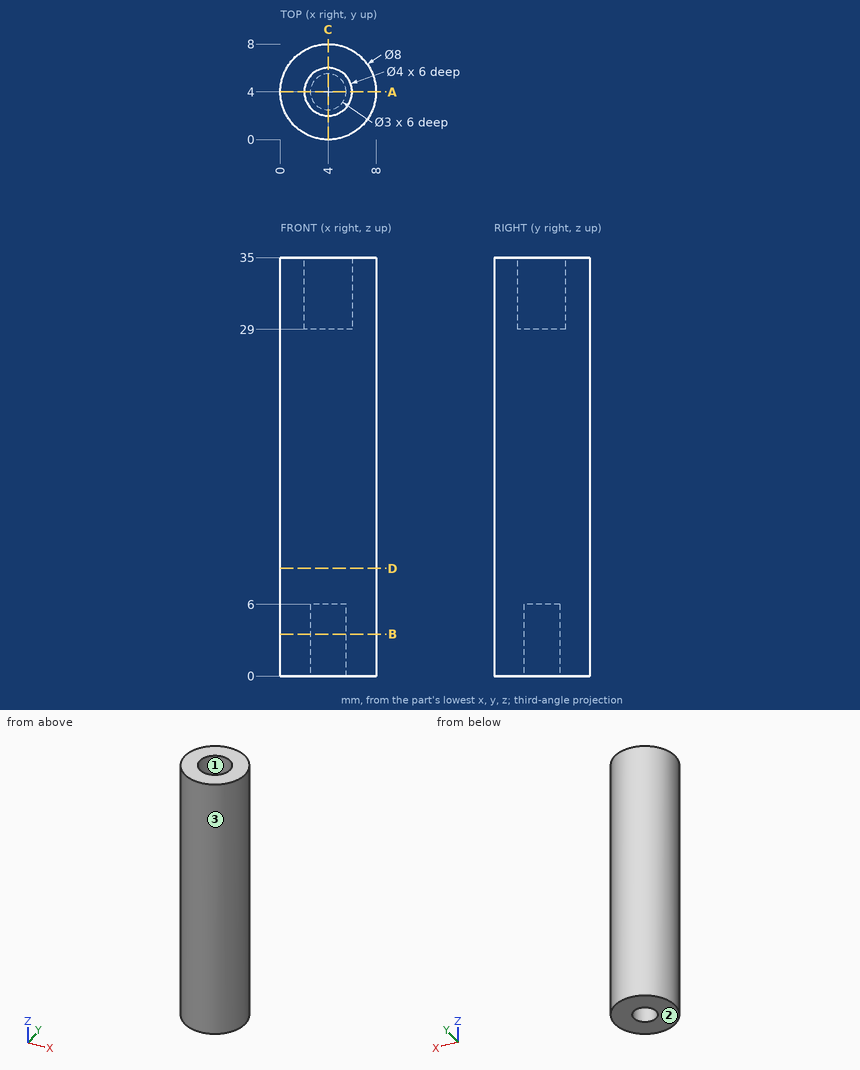
The figure shows three views and two pictorial views of one solid part (mm, origin at its lowest corner). Answer the questions. Give positions to 0.01 mm unless a question says otherwise; leave off trailing zeros. Write each loop counter-clockwise with the first axis right and the second up, starting at its lowest first coordinate (ties: lowest second). Pieces come first, ordered by that corner, then holes. Notation, with made-up numbers: M 12,83 L 56,83 A13 cw 56,105 Z; hole C 89,57.25 d1. An arc over 180 degrees is marked long. Write each question's results on one line, items separated by ' | '.
Q1. Consider L1, parallel to Y at x = 4, z = 33.2; L2, parallel to Y at x = 4, z = 2.75; L3, parallel to Z at x = 3.5, y = 3.75. Determine where each line is inside the solid, lowest interval first. Write a range as from..to.
Output values:
L1: 0..2, 6..8 | L2: 0..2.5, 5.5..8 | L3: 6..29
Q2. Section B-B, the plane z = 3.5 is taken. Write down the section's boundary in (x, y).
Output values:
outline: C 4,4 d8; hole C 4,4 d3
Q3. For a pull along Y with two mould halves and no side action, classify the marked faces 1, 2 and 3 as released by +Y, released by -Y, zero draft, split by the parting line, or undercut.
Output values:
face 1: undercut | face 2: zero draft | face 3: split by the parting line
Q4. A flat-ended cylindrical pin translates along its axis: P1, Ø1.2, axis at x = 3, y = 4, coming from the +Z side. Find the tip coordinate at first contact, or state that the pin passes through.
Output values:
P1: z = 29
Q5. Section A-A, the plane y = 4 is taken. Write down the section's boundary in (x, z), then the cut area to 3 significant figures.
Output values:
outline: M 0,0 L 2.5,0 L 2.5,6 L 5.5,6 L 5.5,0 L 8,0 L 8,35 L 6,35 L 6,29 L 2,29 L 2,35 L 0,35 Z | area: 238 mm2
Q6. Section D-D, the plane z = 9 is taken. Write down the section's boundary in (x, y), then the cut area to 3 significant figures.
Output values:
outline: C 4,4 d8 | area: 50.3 mm2
